For this review, use the dimensioned drawing (mm, ordinates from the lowest corner) and the shaded views. Coordinates: 2 decimals unless noted, no trailing zeros. Write each loop counter-clockwise with the first axis right and the second up, starting at its lowest first coordinate (ties: lowest second). Pieces come first, ordered by that corner, then holes. Notation, with made-up numbers: (71.5, 73) - (115.5, 73) arc R20 ccw to (115.5, 93) - close; hole circle Ø11 at (30.5, 53). An arc over 180 degrees is marked (long way). Use one line per item in the form item = value. Start each with the question number.
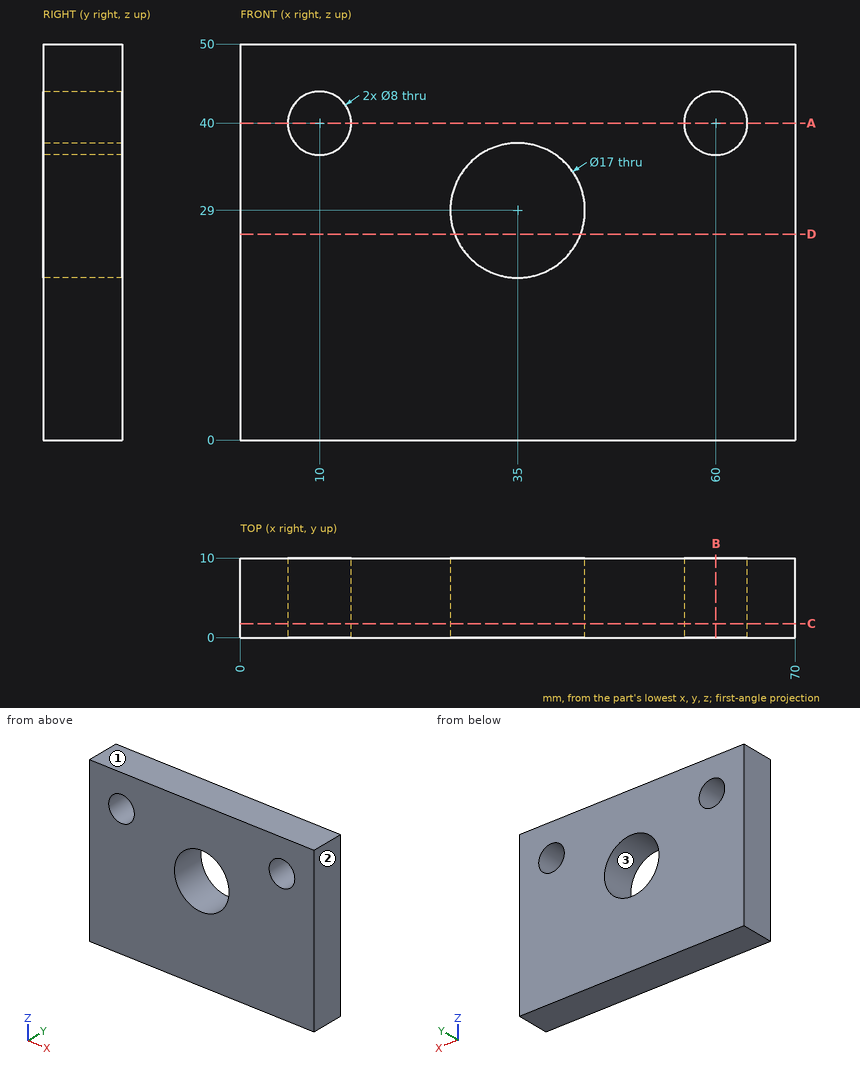
1. Take a section at B-B (x = 60). State the section outline as (y, z) points, plus the area to 3 significant figures.
2. Take a section at C-C (y = 1.75). State the section outline as (x, z) points, plus the area to 3 significant figures.
3. For L1, parallel to Z at x = 35, y = 5.75; L2, parallel to Z at x = 10, y = 6.75; L3, parallel to X at y = 8.5, z = 38, list the stretches that pass through material, from the lowest coordinate up.
4. Take a section at D-D (z = 26). State the section outline as (x, y) points.
5. The part is to be moulded in two halves that separate along X. For the marked faces 1, 2 and 3, say which applies: released by +X, released by -X, zero draft, split by the parting line, or undercut.
6. Take a section at A-A (z = 40). State the section outline as (x, y) points.
Returned:
q1.outline = (0, 0) - (10, 0) - (10, 36) - (0, 36) - close; (0, 44) - (10, 44) - (10, 50) - (0, 50) - close
q1.area = 420 mm²
q2.outline = (0, 0) - (70, 0) - (70, 50) - (0, 50) - close; hole circle Ø8 at (10, 40); hole circle Ø17 at (35, 29); hole circle Ø8 at (60, 40)
q2.area = 3,170 mm²
q3.L1 = 0 to 20.5, 37.5 to 50
q3.L2 = 0 to 36, 44 to 50
q3.L3 = 0 to 6.54, 13.46 to 56.54, 63.46 to 70
q4.outline = (0, 0) - (27.05, 0) - (27.05, 10) - (0, 10) - close; (42.95, 0) - (70, 0) - (70, 10) - (42.95, 10) - close
q5.face_1 = zero draft
q5.face_2 = released by +X
q5.face_3 = undercut
q6.outline = (0, 0) - (6, 0) - (6, 10) - (0, 10) - close; (14, 0) - (56, 0) - (56, 10) - (14, 10) - close; (64, 0) - (70, 0) - (70, 10) - (64, 10) - close
